from build123d import *

# Parameters (mm, degrees)
SKETCH1_R           = 2
BOSS_EXTRUDE1_DEPTH = 25
CUT_EXTRUDE1_REACH  = 108.066
SKETCH2_R           = 8.25
CUT_EXTRUDE2_REACH  = 77
SKETCH3_R           = 6.75


with BuildPart() as part:
    # Sketch1 → Boss-Extrude1 (new body)
    with BuildSketch(Plane(origin=(0, 0, 0), x_dir=(1, 0, 0), z_dir=(0, 1, 0))):
        with BuildLine():
            ThreePointArc((-22, 50), (-24.121320344, 49.121320344), (-25, 47))
            Line((-25, 47), (-25, -47))
            ThreePointArc((-25, -47), (-24.121320344, -49.121320344), (-22, -50))
            Line((-22, -50), (22, -50))
            ThreePointArc((22, -50), (24.121320344, -49.121320344), (25, -47))
            Line((25, -47), (25, 47))
            ThreePointArc((25, 47), (24.121320344, 49.121320344), (22, 50))
            Line((22, 50), (-22, 50))
        make_face()
        with Locations(Location((-22, -47, 0), (0, 0, 270))):
            Circle(SKETCH1_R, mode=Mode.SUBTRACT)
        with BuildLine():
            Line((-22, -44), (-22, 44))
            ThreePointArc((-22, 44), (-19.878679656, 44.878679656), (-19, 47))
            Line((-19, 47), (19, 47))
            ThreePointArc((19, 47), (19.878679656, 44.878679656), (22, 44))
            Line((22, 44), (22, -44))
            ThreePointArc((22, -44), (19.878679656, -44.878679656), (19, -47))
            Line((19, -47), (-19, -47))
            ThreePointArc((-19, -47), (-19.878679656, -44.878679656), (-22, -44))
        make_face(mode=Mode.SUBTRACT)
        with Locations(Location((22, 47, 0), (0, 0, 270))):
            Circle(SKETCH1_R, mode=Mode.SUBTRACT)
        with Locations(Location((-22, 47, 0), (0, 0, 270))):
            Circle(SKETCH1_R, mode=Mode.SUBTRACT)
        with Locations(Location((22, -47, 0), (0, 0, 270))):
            Circle(SKETCH1_R, mode=Mode.SUBTRACT)
    extrude(amount=BOSS_EXTRUDE1_DEPTH)

    # Sketch2 → Cut-Extrude1 (cut, up to next)
    with BuildSketch(Plane.XY.offset(50), mode=Mode.PRIVATE) as cut_extrude1_sk1:
        with Locations((0, 12.5)):
            Circle(SKETCH2_R)
    cut_extrude1_tool1 = extrude(cut_extrude1_sk1.sketch, amount=-CUT_EXTRUDE1_REACH, mode=Mode.PRIVATE) & part.part
    add(cut_extrude1_tool1.solids().sort_by_distance((0, 12.5, 50))[0], mode=Mode.SUBTRACT)

    # Sketch3 → Cut-Extrude2 (cut, up to next)
    with BuildSketch(Plane.ZY.offset(25), mode=Mode.PRIVATE) as cut_extrude2_sk1:
        with Locations((-30, 12.5)):
            Circle(SKETCH3_R)
    cut_extrude2_tool1 = extrude(cut_extrude2_sk1.sketch, amount=-CUT_EXTRUDE2_REACH, mode=Mode.PRIVATE) & part.part
    # Sketch3 → Cut-Extrude2 (cut, up to next)
    with BuildSketch(Plane.ZY.offset(25), mode=Mode.PRIVATE) as cut_extrude2_sk2:
        with Locations((-10, 12.5)):
            Circle(SKETCH3_R)
    cut_extrude2_tool2 = extrude(cut_extrude2_sk2.sketch, amount=-CUT_EXTRUDE2_REACH, mode=Mode.PRIVATE) & part.part
    # Sketch3 → Cut-Extrude2 (cut, up to next)
    with BuildSketch(Plane.ZY.offset(25), mode=Mode.PRIVATE) as cut_extrude2_sk3:
        with Locations((10, 12.5)):
            Circle(SKETCH3_R)
    cut_extrude2_tool3 = extrude(cut_extrude2_sk3.sketch, amount=-CUT_EXTRUDE2_REACH, mode=Mode.PRIVATE) & part.part
    # Sketch3 → Cut-Extrude2 (cut, up to next)
    with BuildSketch(Plane.ZY.offset(25), mode=Mode.PRIVATE) as cut_extrude2_sk4:
        with Locations((30, 12.5)):
            Circle(SKETCH3_R)
    cut_extrude2_tool4 = extrude(cut_extrude2_sk4.sketch, amount=-CUT_EXTRUDE2_REACH, mode=Mode.PRIVATE) & part.part
    add(cut_extrude2_tool1.solids().sort_by_distance((-25, 12.5, -30))[0], mode=Mode.SUBTRACT)
    add(cut_extrude2_tool2.solids().sort_by_distance((-25, 12.5, -10))[0], mode=Mode.SUBTRACT)
    add(cut_extrude2_tool3.solids().sort_by_distance((-25, 12.5, 10))[0], mode=Mode.SUBTRACT)
    add(cut_extrude2_tool4.solids().sort_by_distance((-25, 12.5, 30))[0], mode=Mode.SUBTRACT)


solid = part.part
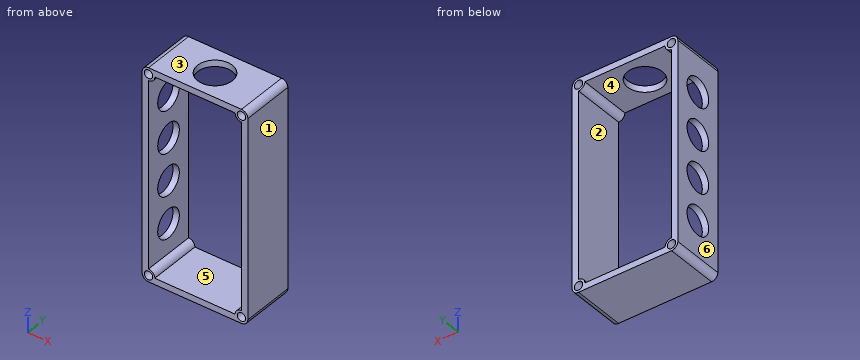
The model under review builds one solid part; all positions refer to its coordinate system, in mm. Face numbers are marked on the shaded views. A direction names the side the tool comes from. Give positions to 0.01 mm unless a question says otherwise; leave off trailing zeros. Order: outer loops, then holes, each group sorted by start corner. A loop starts at its lowest first (then second) coordinate and runs counter-clockwise, first axis right, second up. Notation, with made-up numbers: M 68.25,73.25 L 126.25,73.25 A19 cw 126.25,91.25 Z; hole C 2.5,31 d4. An arc over 180 degrees is marked long. One line per question, with ' | ' between items. Start each with the question number.
1) Wall thickness on L1, parallel to X at y = 10.75, z = 43.5; L2, parallel to Z at x = -8, y = 16; L3, parallel to Y at x = -22.8, z = -30: over which ranges is each line inside the solid? List them lowest first. Write a range as from..to.
2) Consider section A-A, the plane x = -18. Give the boundary of the cut face in (y, z).
3) For the marked faces 1 and 2, list the 3-axis set-ups (+Z, -Z, +X, -X, +Y, -Y) from which the entire face can be reached by the end or side of a thin tool; tool diameter is ignored.
4) Consider section B-B, the plane z = -10. Give the boundary of the cut face in (x, y), then the cut area to 4 significant figures.
5) Consider section D-D, the plane y = 2.75. Give the boundary of the cut face in (x, z).
6) Mouldability with a two-part tool opening along Z and no side actions: class the marked faces 3, 4, 5 and 6 as pulls with the +Z half, pulls with the -Z half, needs draft (parallel to the pull), parting line crosses it, or undercut.
7) Consider section C-C, the plane z = -40. Give the boundary of the cut face in (x, y), then the cut area to 3 significant figures.
8) Clearance check with flat-ended pins moving along their axes: P1, Ø11, axis at y = 12.5, z = -30, coming from the -X side; P2, Ø13, axis at x = 0, y = 12.5, coming from the +Z side. State where each tip first meets the part, or that it passes through.
Found:
1) L1: x = -25..-22, 22..25 | L2: z = -50..-47, 47..50 | L3: y = 0..5.75, 19.25..25
2) outline: M 0,-50 L 25,-50 L 25,-47 L 0,-47 Z; M 0,47 L 25,47 L 25,50 L 0,50 Z
3) face 1: +Z, -Z, +X, +Y, -Y | face 2: +Y, -Y
4) outline: M -25,0 L -22,0 L -22,5.75 L -25,5.75 Z; M -25,19.25 L -22,19.25 L -22,25 L -25,25 Z; M 22,0 L 25,0 L 25,25 L 22,25 Z | area: 109.5 mm²
5) outline: M -25,-47 A3 ccw -22,-50 L 22,-50 A3 ccw 25,-47 L 25,47 A3 ccw 22,50 L -22,50 A3 ccw -25,47 Z; hole C -22,-47 d4; hole C -22,47 d4; hole M -22,-44 A3 cw -19,-47 L 19,-47 A3 cw 22,-44 L 22,44 A3 cw 19,47 L -19,47 A3 cw -22,44 Z; hole C 22,-47 d4; hole C 22,47 d4
6) face 3: pulls with the +Z half | face 4: undercut | face 5: undercut | face 6: needs draft
7) outline: M -25,0 L -22,0 L -22,25 L -25,25 Z; M 22,0 L 25,0 L 25,25 L 22,25 Z | area: 150 mm²
8) P1: stops at x = 22 | P2: stops at z = -47
